Here's the drawing with two shaded views (mm, measured from the low corner). I have some questions. Round coordinates to 2 decimals unless told otherwise and drop trailing zeros. Loops run counter-clockwise (first coordinate to the right, second up) from the corner with the lowest first, then second, coordinate; pieces in that order, holes last. Notation, with made-up numbers: (-1, 16.5) - (46, 16.5) arc R7 cw to (46, 28.5) - close; hole circle Ø5 at (16.25, 34.25). An arc over 180 degrees is marked (long way). Answer as CSV lines item,"result".
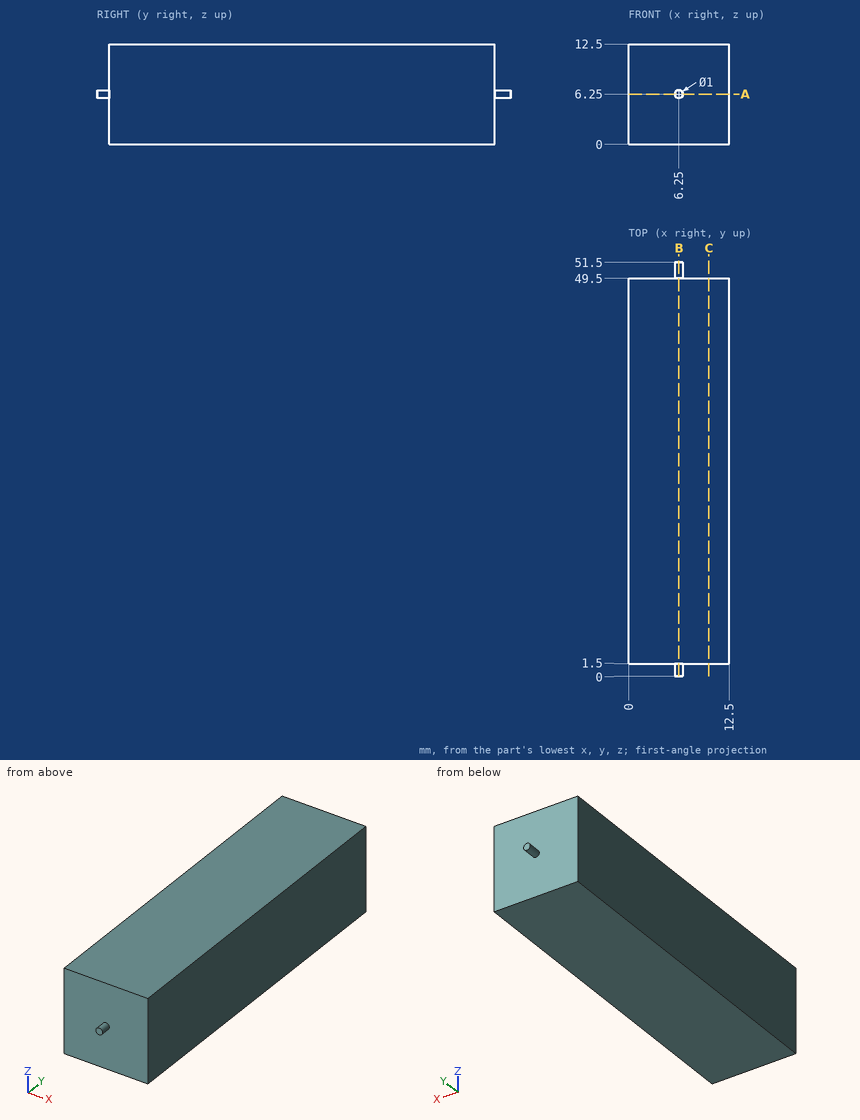
Q1. Imagine slicing it at C-C (x = 10). Write out the boundary of the cut face in (y, z).
Checks:
outline,"(1.5, 0) - (49.5, 0) - (49.5, 12.5) - (1.5, 12.5) - close"
Q2. If I drill on line 1 along Y through (x, z) = (11, 2.75), over which ranges is the centre line in solid material (lowest first)? Write a range as [from, to].
Checks:
line 1,"[1.5, 49.5]"
Q3. I'm going to push flat-ended pins straight in: pin 1 Ø5 at (x, z) = (9.5, 3) entering from +Y; pin 2 Ø6 at (x, z) = (6.5, 10) entering from -Y. Where does each tip first touch, or does it pass through?
Checks:
pin 1,"y = 49.5"
pin 2,"y = 1.5"
Q4. Imagine slicing it at B-B (x = 6.25). Write out the boundary of the cut face in (y, z), then the cut area to 4 significant figures.
Checks:
outline,"(0, 5.75) - (1.5, 5.75) - (1.5, 0) - (49.5, 0) - (49.5, 5.75) - (51.5, 5.75) - (51.5, 6.75) - (49.5, 6.75) - (49.5, 12.5) - (1.5, 12.5) - (1.5, 6.75) - (0, 6.75) - close"
area,"603.5 mm²"
Q5. Imagine slicing it at A-A (z = 6.25). Write out the boundary of the cut face in (x, y).
Checks:
outline,"(0, 1.5) - (5.75, 1.5) - (5.75, 0) - (6.75, 0) - (6.75, 1.5) - (12.5, 1.5) - (12.5, 49.5) - (6.75, 49.5) - (6.75, 51.5) - (5.75, 51.5) - (5.75, 49.5) - (0, 49.5) - close"
